from build123d import *

# Parameters (mm, degrees)
SKETCH1_W           = 27.8
SKETCH1_H           = 15.9
SKETCH1_R           = 1.55
BOSS_EXTRUDE1_DEPTH = 3
SKETCH2_W           = 10.2
SKETCH2_H           = 25
BOSS_EXTRUDE2_DEPTH = 3
SKETCH3_R           = 2.55
CUT_EXTRUDE1_DEPTH  = 3
CUT_EXTRUDE4_START  = -3
SKETCH4_R           = 4.9
SKETCH4_R_2         = 2.55
CUT_EXTRUDE4_DEPTH  = 3


with BuildPart() as part:
    # Sketch1 → Boss-Extrude1 (new body)
    with BuildSketch(Plane(origin=(0, 0, 0), x_dir=(1, 0, 0), z_dir=(0, 1, 0))):
        with Locations((13.9, 7.95)):
            Rectangle(SKETCH1_W, SKETCH1_H)
        with Locations(Location((2.8, 2.8, 0), (0, 0, 270))):
            Circle(SKETCH1_R, mode=Mode.SUBTRACT)
        with Locations(Location((25, 13.1, 0), (0, 0, 270))):
            Circle(SKETCH1_R, mode=Mode.SUBTRACT)
    extrude(amount=BOSS_EXTRUDE1_DEPTH)

    # Sketch2 → Boss-Extrude2 (add)
    with BuildSketch(Plane.XZ):
        with Locations((13.9, -12.5)):
            Rectangle(SKETCH2_W, SKETCH2_H)
    extrude(amount=BOSS_EXTRUDE2_DEPTH)

    # Sketch3 → Cut-Extrude1 (cut)
    with BuildSketch(Plane.XZ.offset(3)):
        with Locations(Location((13.9, -8, 0), (0, 0, 270))):
            Circle(SKETCH3_R)
        with Locations(Location((13.9, -18, 0), (0, 0, 270))):
            Circle(SKETCH3_R)
    extrude(amount=-CUT_EXTRUDE1_DEPTH, mode=Mode.SUBTRACT)

    # Sketch4 → Cut-Extrude4 (cut)
    # profile 1 of 3: a face of its own
    with BuildSketch(Plane(origin=(0, 3, 0), x_dir=(1, 0, 0), z_dir=(0, 1, 0)).offset(CUT_EXTRUDE4_START)):
        with BuildLine():
            Line((18.327188724, 15.9), (15.346547614, 15.9))
            Line((15.346547614, 15.9), (12.453452386, 15.9))
            Line((12.453452386, 15.9), (9.472811276, 15.9))
            ThreePointArc((9.472811276, 15.9), (13.9, 13.1), (18.327188724, 15.9))
        make_face()
    # profile 2 of 3: a face of its own
    with BuildSketch(Plane(origin=(0, 3, 0), x_dir=(1, 0, 0), z_dir=(0, 1, 0)).offset(CUT_EXTRUDE4_START)):
        with Locations(Location((13.9, 8, 0), (0, 0, 270))):
            Circle(SKETCH4_R)
        with Locations(Location((13.9, 8, 0), (0, 0, 90))):
            Circle(SKETCH4_R_2, mode=Mode.SUBTRACT)
    # profile 3 of 3: a face of its own
    with BuildSketch(Plane(origin=(0, 3, 0), x_dir=(1, 0, 0), z_dir=(0, 1, 0)).offset(CUT_EXTRUDE4_START)):
        with Locations(Location((13.9, 8, 0), (0, 0, 90))):
            Circle(SKETCH4_R_2)
    extrude(amount=CUT_EXTRUDE4_DEPTH, mode=Mode.SUBTRACT)


solid = part.part
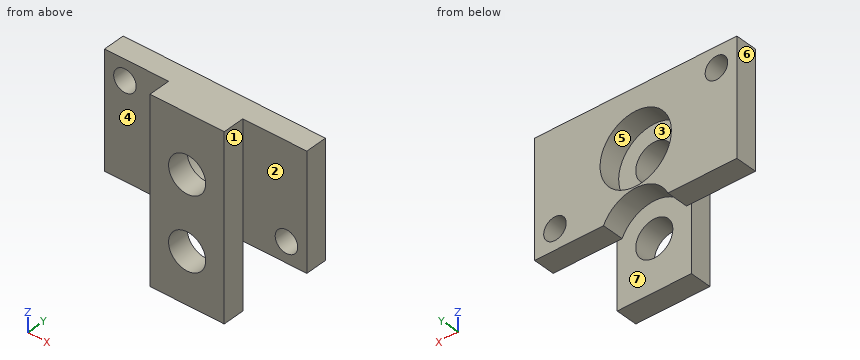
For this review, take the finished solid that the model builds, in its own axes (mm). Face numbers are marked on the shaded views. A direction names the side the tool comes from. Coordinates: 2 decimals unless noted, no trailing zeros. Order: outer loops, then holes, each group sorted by start corner. A loop starts at its lowest first (then second) coordinate and runs counter-clockwise, first axis right, second up. Notation, with made-up numbers: (9, -25) - (31, -25) arc R24 cw to (31, 2) - close; hole circle Ø5 at (25.25, 10.5). An arc over 180 degrees is marked (long way). Use one line per item in the form item = value.
Q1. Consider section B-B (y = 2.65). Give the boundary of the cut face in (x, z).
Checked values:
outline = (0, -15.9) - (9.47, -15.9) arc R4.9 cw to (18.33, -15.9) - (27.8, -15.9) - (27.8, 0) - (0, 0) - close; hole circle Ø3.1 at (2.8, -2.8); hole circle Ø9.8 at (13.9, -8); hole circle Ø3.1 at (25, -13.1)
Q2. Consider section C-C (x = 25). Give the boundary of the cut face in (y, z), then the cut area to 3 significant figures.
Checked values:
outline = (0, -15.9) - (3, -15.9) - (3, -14.65) - (0, -14.65) - close; (0, -11.55) - (3, -11.55) - (3, 0) - (0, 0) - close
area = 38.4 mm2
Q3. Draft analysis for pull direction X (two halves, no side actions). For the marked faces 1, 2 and 3, state which applies: +X half, -X half, draft (parallel to the pull), parting line (faces both ways), or undercut.
Checked values:
face_1 = +X half
face_2 = draft
face_3 = undercut
Q4. For P1, Ø8, axis at x = 13.9, z = -8, coming from the +Y side; P2, Ø3, axis at x = 21.5, z = -14.5, coming from the -Y side; P3, Ø0.9, axis at y = -1.5, z = -15.5, coming from the +X side; P4, Ø3, axis at x = 2.8, z = -2.8, coming from the +Y side, all flat-tipped, find the tip position at first contact; note any pin that passes through.
Checked values:
P1 = 0
P2 = 0
P3 = 19
P4 = through
Q5. For the marked faces 4, 5, 6 and 7, list the 3-axis set-ups (+Z, -Z, +X, -X, +Y, -Y) from which the entire face can be reached by the end or side of a thin tool; tool diameter is ignored.
Checked values:
face_4 = +Z, -Z, -X, -Y
face_5 = +Y
face_6 = +Z, -Z, -X, +Y, -Y
face_7 = -Z, +Y
Q6. For probe 1 along X at (y, z) = (-1.4, -18); probe 2 along Y at (x, z) = (24.5, -15.25); probe 3 along X at (y, z) = (2.55, -2.75), list the stretches that pass through material, from the lowest coordinate up. Write a range as from..to.
Checked values:
probe_1 = 8.8..11.35, 16.45..19
probe_2 = 0..3
probe_3 = 0..1.25, 4.35..27.8
Q7. Consider section D-D (x = 13.9). Give the boundary of the cut face in (y, z).
Checked values:
outline = (-3, -25) - (0, -25) - (0, -20.55) - (-3, -20.55) - close; (-3, -15.45) - (0, -15.45) - (0, -13.1) - (3, -13.1) - (3, -12.9) - (0, -12.9) - (0, -10.55) - (-3, -10.55) - close; (-3, -5.45) - (0, -5.45) - (0, -3.1) - (3, -3.1) - (3, 0) - (-3, 0) - close
Q8. Consider section A-A (z = -8). Give the boundary of the cut face in (x, y).
Checked values:
outline = (0, 0) - (8.8, 0) - (8.8, -3) - (11.35, -3) - (11.35, 0) - (9, 0) - (9, 3) - (0, 3) - close; (16.45, -3) - (19, -3) - (19, 0) - (27.8, 0) - (27.8, 3) - (18.8, 3) - (18.8, 0) - (16.45, 0) - close
